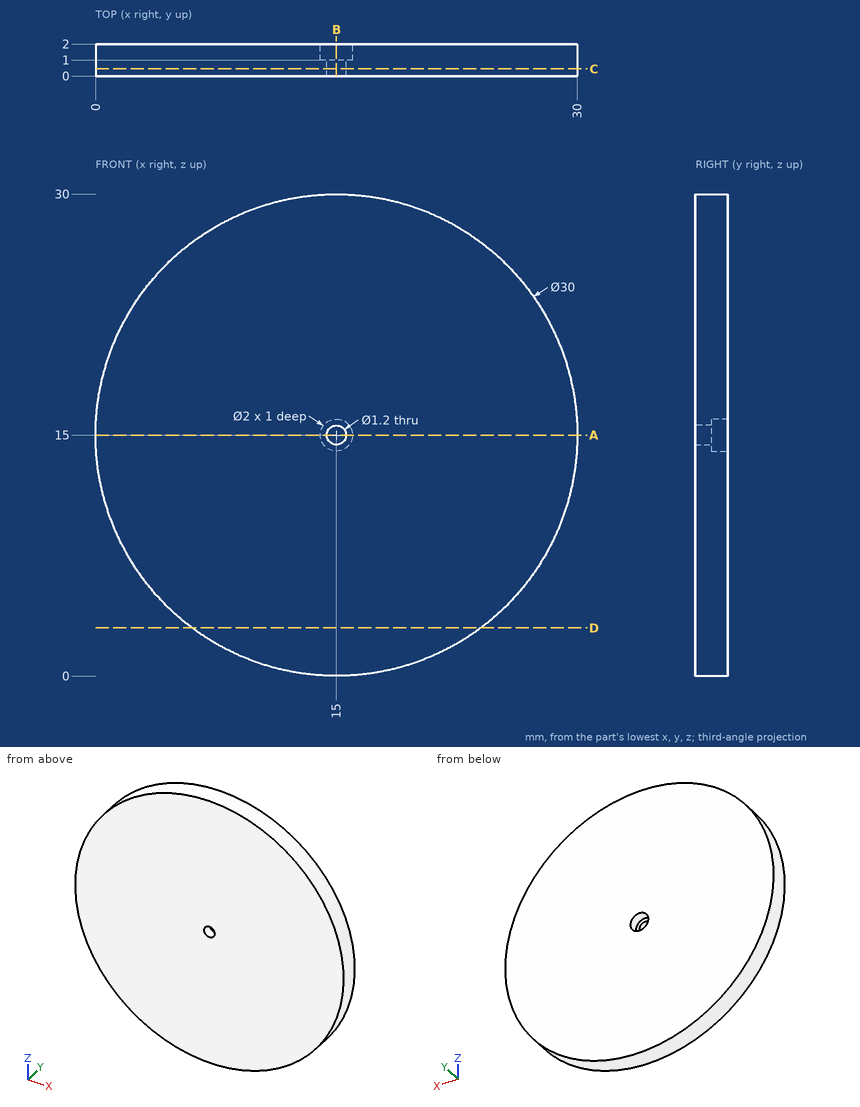
Here's the drawing with two shaded views (mm, measured from the low corner). I have some questions. Coordinates: 2 decimals unless noted, no trailing zeros. Write each loop counter-clockwise with the first axis right and the second up, starting at its lowest first coordinate (ties: lowest second). Pieces come first, ordered by that corner, then holes. Notation, with made-up numbers: (-28, 83) - (-3, 83) arc R22 cw to (-3, 98) - close; hole circle Ø8 at (-22.5, 5). An arc over 180 degrees is marked (long way). Return JSON: item names as keys, results as strings.
Q1. If we section it at A-A (z = 15): Please give me the cut outline in (x, y), then the cut area to 3 significant figures.
Computed values:
{"outline": "(0, 0) - (14.4, 0) - (14.4, 1) - (14, 1) - (14, 2) - (0, 2) - close; (15.6, 0) - (30, 0) - (30, 2) - (16, 2) - (16, 1) - (15.6, 1) - close", "area": "56.8 mm2"}
Q2. I'm going to push a flat-ended pin straight in: pin 1 Ø1.1 at (x, z) = (15, 15) entering from +Y. Where does the tip first touch, or does it pass through?
Computed values:
{"pin 1": "passes through"}
Q3. Please list where these lines run through material, in increasing order: L1, parallel to X at y = 0.6, z = 15; L2, parallel to X at y = 1.45, z = 15; L3, parallel to Z at x = 21.75, y = 1. Write a range as from..to.
Computed values:
{"L1": "x = 0..14.4, 15.6..30", "L2": "x = 0..14, 16..30", "L3": "z = 1.6..28.4"}
Q4. If we section it at B-B (x = 15): Please give me the cut outline in (y, z).
Computed values:
{"outline": "(0, 0) - (2, 0) - (2, 14) - (1, 14) - (1, 14.4) - (0, 14.4) - close; (0, 15.6) - (1, 15.6) - (1, 16) - (2, 16) - (2, 30) - (0, 30) - close"}
Q5. If we section it at D-D (z = 3): Please give me the cut outline in (x, y).
Computed values:
{"outline": "(6, 0) - (24, 0) - (24, 2) - (6, 2) - close"}
Q6. If we section it at C-C (y = 0.45): Please give me the cut outline in (x, z).
Computed values:
{"outline": "circle Ø30 at (15, 15); hole circle Ø1.2 at (15, 15)"}
